The model under review builds one solid part; all positions refer to its coordinate system, in mm. Face numbers are marked on the shaded views. A direction names the side the tool comes from. Round coordinates to 2 decimals unless told otherwise and drop trailing zeros. Order: outer loops, then holes, each group sorted by start corner. A loop starts at its lowest first (then second) coordinate and runs counter-clockwise, first axis right, second up. Notation, with made-up numbers: (74, 35.25) -> (88, 35.25) arc R14 ccw to (88, 54.25) -> close; hole circle Ø1 at (10.5, 59). An arc over 180 degrees is marked (long way). Return JSON: item names as keys, results as strings. Group by question number.
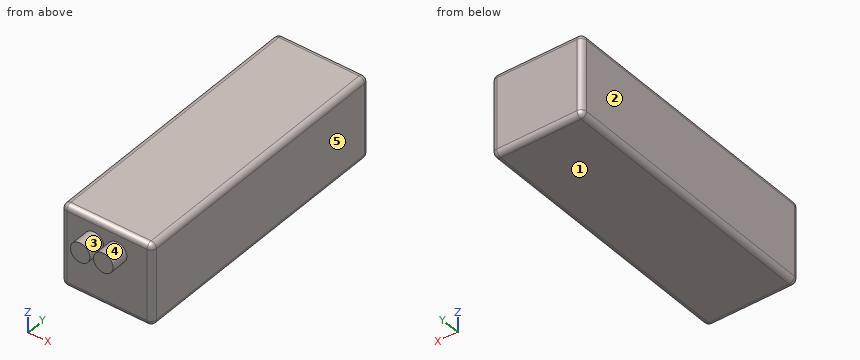
from build123d import *

# Parameters (mm, degrees)
SKETCH1_W           = 51
SKETCH1_H           = 46
BOSS_EXTRUDE1_DEPTH = 156
FILLET1_R           = 3
SKETCH2_R           = 5.479665814
BOSS_EXTRUDE2_DEPTH = 10


with BuildPart() as part:
    # Sketch1 → Boss-Extrude1 (new body)
    with BuildSketch(Plane(origin=(0, 0, 0), x_dir=(1, 0, 0), z_dir=(0, 1, 0))):
        with Locations((-13.995554746, -2.3)):
            Rectangle(SKETCH1_W, SKETCH1_H)
    extrude(amount=BOSS_EXTRUDE1_DEPTH)

    # Fillet1
    fillet1_edges = [part.edges().sort_by_distance(p)[0] for p in [
        (11.504445254, 156, 2.3),
        (-13.995554746, 156, -20.7),
        (-39.495554746, 156, 2.3),
        (-13.995554746, 0, -20.7),
        (11.504445254, 0, 2.3),
        (-13.995554746, 0, 25.3),
        (-39.495554746, 0, 2.3),
        (-39.495554746, 78, -20.7),
        (11.504445254, 78, -20.7),
        (11.504445254, 78, 25.3),
        (-39.495554746, 78, 25.3),
        (-13.995554746, 156, 25.3),
    ]]
    fillet(fillet1_edges, radius=FILLET1_R)

    # Sketch2 → Boss-Extrude2 (add)
    with BuildSketch(Plane.XZ):
        with Locations((-21.241241136, 12.3252816)):
            Circle(SKETCH2_R)
        with Locations((-8.248975885, 12.82498411)):
            Circle(SKETCH2_R)
    extrude(amount=BOSS_EXTRUDE2_DEPTH)


solid = part.part
Item 1: Consider section B-B on x = 5. State the section outline as (y, z) points, plus the area to 3 significant figures.
Item 2: Insertion check: pin 1 Ø8 at (x, z) = (-22, -1) entering from -Y. The pin has a flat end and moves straight along its axis. Give the tip position at first contact, or say it passes through.
Item 3: The part is to be moulded in two halves that separate along X. For the marked faces 1, 2 and 3, say which applies: +X half, -X half, draft (parallel to the pull), parting line (faces both ways), or undercut.
Item 4: Consider section C-C on x = -24.5. State the section outline as (y, z) points, plus the area to 3 significant figures.
Item 5: Consider section D-D on x = -6.5. State the section outline as (y, z) points.
Item 6: Consider section A-A on z = -12.5. State the section outline as (x, y) points, plus the area to 3 significant figures.
Item 7: For the marked faces 4 and 5, list the 3-axis set-ups (+Z, -Z, +X, -X, +Y, -Y) from which the entire face can be reached by the end or side of a thin tool; tool diameter is ignored.
Item 8: Wall thickness on line 1 along Y through (x, z) = (-13, -8); line 2 along Z through (x, y) = (-37, 29): over which ranges is each line inside the solid? List them lowest first.
Values:
{
 "1": {"outline": "(0, -17.7) arc R3 ccw to (3, -20.7) -> (153, -20.7) arc R3 ccw to (156, -17.7) -> (156, 22.3) arc R3 ccw to (153, 25.3) -> (3, 25.3) arc R3 ccw to (0, 22.3) -> close", "area": "7,170 mm^2"},
 "2": {"pin 1": "y = 0"},
 "3": {"face 1": "draft", "face 2": "-X half", "face 3": "undercut"},
 "4": {"outline": "(-10, 7.92) -> (0, 7.92) -> (0, -17.7) arc R3 ccw to (3, -20.7) -> (153, -20.7) arc R3 ccw to (156, -17.7) -> (156, 22.3) arc R3 ccw to (153, 25.3) -> (3, 25.3) arc R3 ccw to (0, 22.3) -> (0, 16.73) -> (-10, 16.73) -> close", "area": "7,260 mm^2"},
 "5": {"outline": "(-10, 7.63) -> (0, 7.63) -> (0, -17.7) arc R3 ccw to (3, -20.7) -> (153, -20.7) arc R3 ccw to (156, -17.7) -> (156, 22.3) arc R3 ccw to (153, 25.3) -> (3, 25.3) arc R3 ccw to (0, 22.3) -> (0, 18.02) -> (-10, 18.02) -> close"},
 "6": {"outline": "(-39.5, 3) arc R3 ccw to (-36.5, 0) -> (8.5, 0) arc R3 ccw to (11.5, 3) -> (11.5, 153) arc R3 ccw to (8.5, 156) -> (-36.5, 156) arc R3 ccw to (-39.5, 153) -> close", "area": "7,950 mm^2"},
 "7": {"face 4": "-Y", "face 5": "+Z, -Z, +X, +Y, -Y"},
 "8": {"line 1": "0 to 156", "line 2": "-20.66 to 25.26"}
}
